Geometry: see drawing. Coordinates: mm, zero at the bounding-box minimum. A direction names the side the tool comes from. Coordinates: 2 decimals unless noted, no trailing zeros. Order: outer loops, then holes, each group sorted by start corner. A loop starts at its lowest first (then second) coordinate and runs counter-clockwise, first axis right, second up. Notation, with made-up numbers: M 39,-16.5 L 45,-16.5 A9 cw 45,-0.5 Z; hole C 39.25,40 d4. An arc over 180 degrees is marked long. Answer in a Markdown table with one row per item.
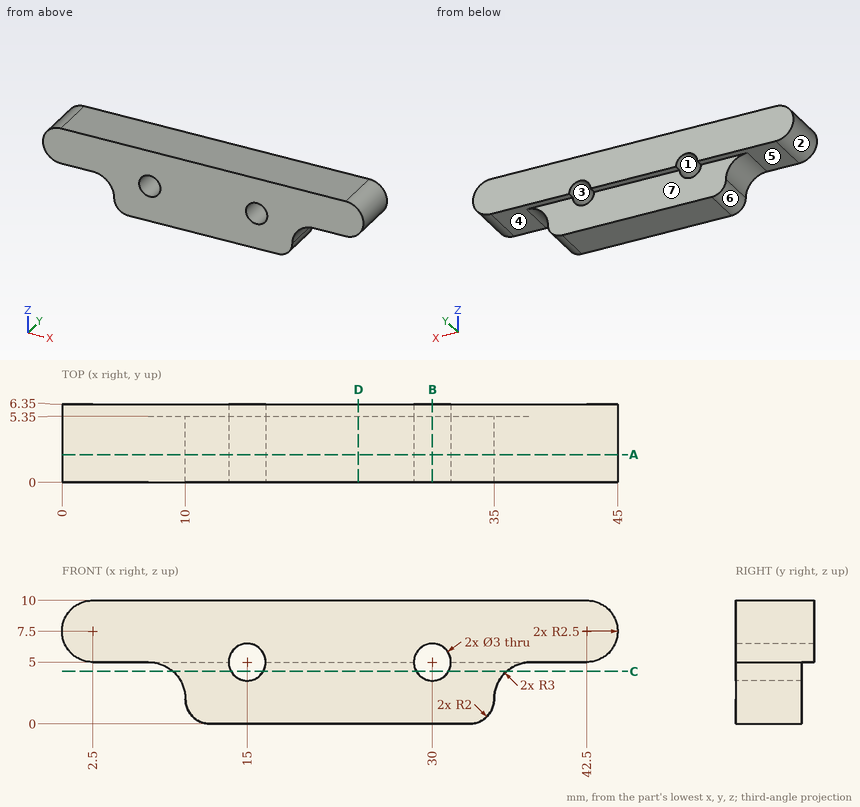
1) Cut plane B-B, the plane x = 30. Output: boundary loops of the cut face in (y, z).
Resolved:
| item | result |
|---|---|
| outline | M 0,0 L 5.35,0 L 5.35,3.5 L 0,3.5 Z; M 0,6.5 L 6.35,6.5 L 6.35,10 L 0,10 Z |
2) Mould query, pull axis X, two halves, no side actions, for the marked faces 1, 2, 3 and 4. Classes: +X half, -X half, draft (parallel to the pull), parting line (faces both ways), or undercut.
Resolved:
| item | result |
|---|---|
| face 1 | undercut |
| face 2 | -X half |
| face 3 | undercut |
| face 4 | draft |
3) Cut plane D-D, the plane x = 24. Output: boundary loops of the cut face in (y, z).
Resolved:
| item | result |
|---|---|
| outline | M 0,0 L 5.35,0 L 5.35,5 L 6.35,5 L 6.35,10 L 0,10 Z |
4) Contact query for flat-ended pins moving along their axis: pin 1 (1.5 mm diameter, centred on x = 37.5, z = 4, fed in from +Y); pin 2 (0.5 mm diameter, centred on x = 21, y = 6, fed in from -Z). Output: stop coordinate, or through.
Resolved:
| item | result |
|---|---|
| pin 1 | passes through |
| pin 2 | stops at z = 5 |
5) Cut plane C-C, the plane z = 4.25. Output: boundary loops of the cut face in (x, y), and give its area (3 significant figures).
Resolved:
| item | result |
|---|---|
| outline | M 8.98,0 L 13.7,0 L 13.7,5.35 L 8.98,5.35 Z; M 16.3,0 L 28.7,0 L 28.7,5.35 L 16.3,5.35 Z; M 31.3,0 L 36.02,0 L 36.02,5.35 L 31.3,5.35 Z |
| area | 117 mm2 |
6) Material intervals for probe 1 along Z at (x, y) = (15, 2.5); probe 2 along X at (y, z) = (6, 6); probe 3 along X at (y, z) = (4.75, 6.25) (1 decimal), sorted ascending.
Resolved:
| item | result |
|---|---|
| probe 1 | z = 0 to 3.5, 6.5 to 10 |
| probe 2 | x = 0.5 to 13.88, 16.12 to 28.88, 31.12 to 44.5 |
| probe 3 | x = 0.3 to 14.2, 15.8 to 29.2, 30.8 to 44.7 |
7) Reachability of the marked faces 5, 6 and 7 from +Z, -Z, +X, -X, +Y, -Y: full face, straight path, thin tool, end or side. Return the list, or none.
Resolved:
| item | result |
|---|---|
| face 5 | -Z, -X, +Y |
| face 6 | -Z, -X, +Y, -Y |
| face 7 | -Z, +X, -X, +Y |
8) Cut plane A-A, the plane y = 2.25. State how many separate pieces and enclosed holes the cut face has, and give its area (3 significant figures).
Resolved:
| item | result |
|---|---|
| separate pieces | 1 |
| enclosed holes | 2 |
| area | 333 mm2 |
